from build123d import *

# Parameters (mm, degrees)
SALIENTE_EXTRUIR1_DEPTH            = 8
CROQUIS2_W                         = 3
CROQUIS2_H                         = 7
CORTAR_EXTRUIR1_DEPTH              = 10
CORTAR_EXTRUIR3_REACH              = 35.619
CROQUIS3_R                         = 1.5
CORTAR_EXTRUIR3_DIRECTION_2_REACH  = 35.619
CROQUIS6_W                         = 10
CROQUIS6_H                         = 7
CORTAR_REVOLUCI_N4_ANGLE           = 130
CORTAR_REVOLUCI_N4_OTHER_WAY_ANGLE = 60
CROQUIS7_R                         = 0.5
CORTAR_EXTRUIR4_DEPTH              = 10


with BuildPart() as part:
    # Croquis1 → Saliente-Extruir1 (new body)
    with BuildSketch(Plane.XY):
        with BuildLine():
            Line((-5, 31.606961259), (-5, 24.5))
            Line((-5, 24.5), (5, 24.5))
            Line((5, 24.5), (5, 31.606961259))
            ThreePointArc((5, 31.606961259), (0, 32), (-5, 31.606961259))
        make_face()
    extrude(amount=SALIENTE_EXTRUIR1_DEPTH)

    # Croquis2 → Cortar-Extruir1 (cut)
    with BuildSketch(Plane.XZ.offset(-24.5)):
        with Locations((0, 4.5)):
            Rectangle(CROQUIS2_W, CROQUIS2_H)
    extrude(amount=-CORTAR_EXTRUIR1_DEPTH, mode=Mode.SUBTRACT)

    # Cortar-Extruir3: up to this face of the body (flat: up to its plane)
    cortar_extruir3_end = Plane(part.part.faces().sort_by_distance((-5, 28.053480629, 4))[0])
    # Croquis3 → Cortar-Extruir3 (cut, up to the picked face)
    with BuildSketch(Plane(origin=(-1.5, 0, 0), x_dir=(0, 0, -1), z_dir=(1, 0, 0)), mode=Mode.PRIVATE) as cortar_extruir3_sk1:
        with Locations((-5, 28.232412208)):
            Circle(CROQUIS3_R)
    cortar_extruir3_tool1 = split(extrude(cortar_extruir3_sk1.sketch, amount=-CORTAR_EXTRUIR3_REACH, mode=Mode.PRIVATE), bisect_by=cortar_extruir3_end, keep=Keep.BOTH, mode=Mode.PRIVATE)
    add(cortar_extruir3_tool1.solids().sort_by(Axis((-1.5, 28.232412, 5), (-1, 0, 0)))[0], mode=Mode.SUBTRACT)

    # Cortar-Extruir3 direction 2: up to this face of the body (flat: up to its plane)
    cortar_extruir3_direction_2_end = Plane(part.part.faces().sort_by_distance((5, 28.053480629, 4))[0])
    # Croquis3 → Cortar-Extruir3 direction 2 (cut, up to the picked face)
    with BuildSketch(Plane(origin=(-1.5, 0, 0), x_dir=(0, 0, -1), z_dir=(1, 0, 0)), mode=Mode.PRIVATE) as cortar_extruir3_direction_2_sk1:
        with Locations((-5, 28.232412208)):
            Circle(CROQUIS3_R)
    cortar_extruir3_direction_2_tool1 = split(extrude(cortar_extruir3_direction_2_sk1.sketch, amount=CORTAR_EXTRUIR3_DIRECTION_2_REACH, mode=Mode.PRIVATE), bisect_by=cortar_extruir3_direction_2_end, keep=Keep.BOTH, mode=Mode.PRIVATE)
    add(cortar_extruir3_direction_2_tool1.solids().sort_by(Axis((-1.5, 28.232412, 5), (1, 0, 0)))[0], mode=Mode.SUBTRACT)

    # Croquis6 → Cortar-Revolución4 (revolve, cut)
    with BuildSketch(Plane(origin=(0, 28.232412208, 0), x_dir=(1, 0, 0), z_dir=(0, 1, 0))):
        with Locations((0, -11.5)):
            Rectangle(CROQUIS6_W, CROQUIS6_H)
    revolve(axis=Axis((1.5, 28.232412208, 5), (1, 0, 0)), revolution_arc=CORTAR_REVOLUCI_N4_ANGLE, mode=Mode.SUBTRACT)

    # Croquis6 → Cortar-Revolución4 other way (revolve, cut)
    with BuildSketch(Plane(origin=(0, 28.232412208, 0), x_dir=(1, 0, 0), z_dir=(0, 1, 0))):
        with Locations((0, -11.5)):
            Rectangle(CROQUIS6_W, CROQUIS6_H)
    revolve(axis=Axis((1.5, 28.232412208, 5), (-1, 0, 0)), revolution_arc=CORTAR_REVOLUCI_N4_OTHER_WAY_ANGLE, mode=Mode.SUBTRACT)

    # Croquis7 → Cortar-Extruir4 (cut)
    with BuildSketch(Plane.XY.offset(1)):
        with Locations((0, 29)):
            Circle(CROQUIS7_R)
    extrude(amount=-CORTAR_EXTRUIR4_DEPTH, mode=Mode.SUBTRACT)


solid = part.part
The model under review builds one solid part; all positions refer to its coordinate system, in mm. A direction names the side the tool comes from. Round coordinates to 2 decimals unless told otherwise and drop trailing zeros. Order: outer loops, then holes, each group sorted by start corner. A loop starts at its lowest first (then second) coordinate and runs counter-clockwise, first axis right, second up. Notation, with made-up numbers: (43.25, 77.5) -> (84.25, 77.5) arc R27 ccw to (84.25, 99.5) -> close; hole circle Ø9 at (12, 10). An arc over 180 degrees is marked (long way). Use CSV: the item, a comma, the result in double quotes. Start each with the question number.
(1) Mouldability with a two-part tool opening along X and no side actions: class faces 4 (the face through (5, 29, 3)), 5 (the face through (-3.274, 31.39, 6.823)), 6 (the face through (1.5, 28, 3)), 7 (the face through (2.3, 31.917, 3.527)) as pulls with the +X half, pulls with the -X half, needs draft (parallel to the pull), parting line crosses it, or undercut.
(2) Insertion check: pin 1 (1.8 mm diameter, centred on y = 28.23, z = 5, fed in from -X); pin 2 (1.5 mm diameter, centred on x = 0.5, y = 30, fed in from +Z); pin 3 (3.5 mm diameter, centred on y = 27, z = 5.5, fed in from +X). Each pin has a flat end and moves straight along its axis. Give the tip position at first contact, or say it passes through.
(3) Consider section A-A on x = 0. Write out the cut boundary in (y, z).
(4) Wall thickness on probe 1 along X at (y, z) = (26.75, 3); probe 2 along Z at (x, y) = (0.25, 27.75); probe 3 along Y at (x, z) = (-3.95, 5): over which ranges is each line inside the solid? List them lowest first. Write a range as from..to.
(5) Tool access review of faces 1 (the face through (-1.5, 28, 3)), 2 (the face through (-3.27, 25.23, 2.48)), 3 (the face through (3.225, 31.39, 6.823)): name each direction out of +Z, -Z, +X, -X, +Y, -Y from which nothing blocks a thin tool from reaching the whole face with its end or side.
(6) Consider section B-B on z = 5. Write out the cut boundary in (x, y), and give its area (3 significant figures).
(7) Consider section D-D on y = 29. Write out the cut boundary in (x, z).
(8) Consider section C-C on x = 3.75. Write out the cut boundary in (y, z).
Responses:
1,face 4,"pulls with the +X half"
1,face 5,"needs draft"
1,face 6,"undercut"
1,face 7,"parting line crosses it"
2,pin 1,"through"
2,pin 2,"z = 1"
2,pin 3,"x = 5"
3,outline,"(24.5, 0) -> (28.5, 0) -> (28.5, 1) -> (24.5, 1) -> close; (29.5, 0) -> (32, 0) -> (32, 1) -> (29.5, 1) -> close"
4,probe 1,"-5..-1.5, 1.5..5"
4,probe 2,"0..1"
4,probe 3,"25.23..26.73, 29.73..31.76"
5,face 1,"+Z, +Y, -Y"
5,face 2,"+X, -X, -Y"
5,face 3,"+Z, +X, -X"
6,outline,"(-5, 25.23) -> (-1.5, 25.23) -> (-1.5, 26.73) -> (-5, 26.73) -> close; (-5, 29.73) -> (-1.5, 29.73) -> (-1.5, 31.96) arc R32 ccw to (-5, 31.61) -> close; (1.5, 25.23) -> (5, 25.23) -> (5, 26.73) -> (1.5, 26.73) -> close; (1.5, 29.73) -> (5, 29.73) -> (5, 31.61) arc R32 ccw to (1.5, 31.96) -> close"
6,area,"25.1 mm²"
7,outline,"(-5, 0) -> (-0.5, 0) -> (-0.5, 1) -> (-1.5, 1) -> (-1.5, 3.71) -> (-5, 3.71) -> close; (-5, 6.29) -> (-1.5, 6.29) -> (-1.5, 7.9) -> (-5, 7.9) -> close; (0.5, 0) -> (5, 0) -> (5, 3.71) -> (1.5, 3.71) -> (1.5, 1) -> (0.5, 1) -> close; (1.5, 6.29) -> (5, 6.29) -> (5, 7.9) -> (1.5, 7.9) -> close"
8,outline,"(24.5, 0) -> (31.78, 0) -> (31.78, 7.05) -> (30.83, 6.5) arc R3 ccw (long way) to (25.93, 3.07) -> (24.5, 1.87) -> close; hole circle Ø3 at (28.23, 5)"
